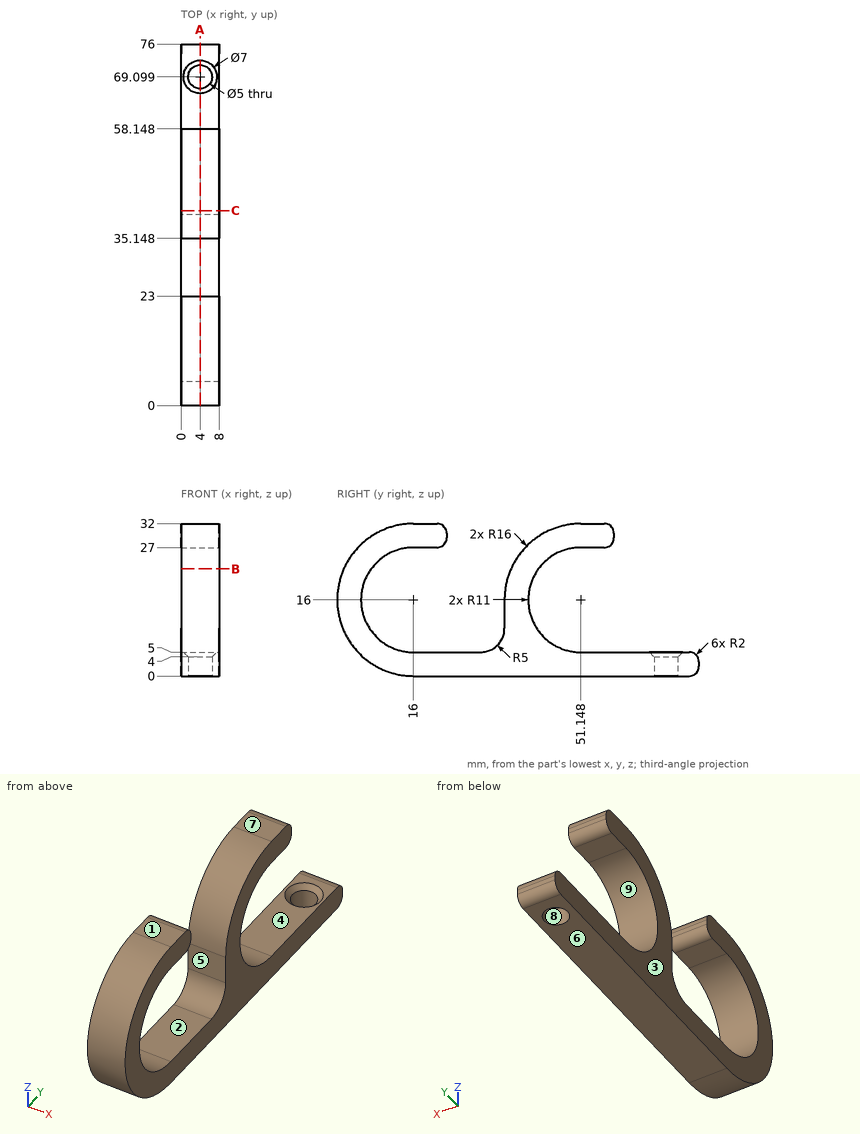
Can you work these out from the drawing? Everything is in mm from the part's minimum corner. A direction names the side the tool comes from. Round coordinates to 2 decimals unless told otherwise and drop trailing zeros. Loops run counter-clockwise (first coordinate to the right, second up) from the corner with the lowest first, then second, coordinate; pieces in that order, holes last. Notation, with made-up numbers: (67, 22.25) - (88, 22.25) arc R13 ccw to (88, 26.25) - close; hole circle Ø4 at (42, -25.75). An arc over 180 degrees is marked (long way). Answer as CSV lines item,"result".
1. I want a section at C-C on y = 41. List the corners of the cut face in (x, z) for me (1 decimal), then the cut area to 3 significant figures.
Filled in:
outline,"(0, 0) - (8, 0) - (8, 11.8) - (0, 11.8) - close; (0, 20.2) - (8, 20.2) - (8, 28.4) - (0, 28.4) - close"
area,"159 mm^2"
2. On a 3-axis mill with a long thin cutter (end or side, diameter ignored), from which of +Z, -Z, +X, -X, +Y, -Y can I reach the whole of each face in a straight line? I mean the marked faces 1, 2, 3, 4 and 5. Say none if no direction works.
Filled in:
face 1,"+Z, +X, -X, +Y, -Y"
face 2,"+X, -X"
face 3,"+Z, -Z, -X, +Y, -Y"
face 4,"+X, -X, +Y"
face 5,"+Z, +X, -X"
3. Please list where these lines run through material, in increasing order: line 1 along Z through (x, y) = (4.5, 55); line 2 along X through (y, z) = (69, 3.5); line 3 along Z through (x, y) = (4, 24). Write a range as [from, to].
Filled in:
line 1,"z = [0, 5], [27, 32]"
line 2,"x = [0, 1.5], [6.5, 8]"
line 3,"z = [0, 5]"
4. I want a section at A-A on x = 4. List the corners of the cut face in (y, z) for me, then the cut area to 3 significant figures.
Filled in:
outline,"(16, 0) - (66.6, 0) - (66.6, 4) - (65.6, 5) - (51.15, 5) arc R11 cw to (51.15, 27) - (56.15, 27) arc R2 ccw to (58.15, 29) - (58.15, 30) arc R2 ccw to (56.15, 32) - (51.15, 32) arc R16 ccw to (35.15, 16) - (35.15, 10) arc R5 cw to (30.15, 5) - (16, 5) arc R11 cw to (16, 27) - (21, 27) arc R2 ccw to (23, 29) - (23, 30) arc R2 ccw to (21, 32) - (16, 32) arc R16 ccw to start; (71.6, 0) - (74, 0) arc R2 ccw to (76, 2) - (76, 3) arc R2 ccw to (74, 5) - (72.6, 5) - (71.6, 4) - close"
area,"743 mm^2"
5. I want a section at B-B on z = 22.5. List the corners of the cut face in (x, y) for me.
Filled in:
outline,"(0, 1.38) - (8, 1.38) - (8, 7.13) - (0, 7.13) - close; (0, 36.53) - (8, 36.53) - (8, 42.27) - (0, 42.27) - close"
6. We'd pull the mould along Z, two halves only. Please class the marked faces 6, 7, 8 and 9: +Z half, -Z half, draft (parallel to the pull), parting line (faces both ways), or undercut.
Filled in:
face 6,"-Z half"
face 7,"+Z half"
face 8,"draft"
face 9,"undercut"
7. For pin 1 Ø4.5 at (x, y) = (4, 69.099) entering from +Z; pin 2 Ø2 at (x, z) = (5.5, 5) entering from -Y; pin 3 Ø0.5 at (x, z) = (2, 29.5) entering from +Y; pin 4 Ø1 at (x, z) = (2.5, 15) entering from -Y, each with a flat end and sliding along its axis, tell me the tip position at first contact or that it passes through.
Filled in:
pin 1,"passes through"
pin 2,"stops at y = 3.51"
pin 3,"stops at y = 58.15"
pin 4,"stops at y = 0.01"
